Could you check a few things on this model? Use its own coordinates, in mm. A direction names the side the tool comes from. Round coordinates to 2 decimals unless told otherwise and drop trailing zeros. Loops run counter-clockwise (first coordinate to the right, second up) from the corner with the lowest first, then second, coordinate; pieces in that order, holes last. Notation, with made-up numbers: (40.5, 18) -> (92.5, 18) arc R32 ccw to (92.5, 50) -> close; hole circle Ø5 at (62.5, -23.5). An arc over 180 degrees is marked (long way). One line per item, written item: value.
from build123d import *

# Parameters (mm, degrees)
SKETCH1_R           = 27.5
SKETCH1_R_2         = 25
BOSS_EXTRUDE1_DEPTH = 100
SKETCH1_4_R         = 25
BOSS_EXTRUDE2_DEPTH = 175
BOSS_EXTRUDE4_START = 95
SKETCH6_R           = 27.5
SKETCH6_R_2         = 25
BOSS_EXTRUDE4_DEPTH = 95
BOSS_EXTRUDE5_START = 90
SKETCH8_R           = 25
BOSS_EXTRUDE5_DEPTH = 90
CUT_EXTRUDE1_START  = -115.215
CUT_EXTRUDE1_DEPTH  = 100.215
CUT_EXTRUDE3_START  = -40
SKETCH10_R          = 25
CUT_EXTRUDE3_DEPTH  = 40
CUT_EXTRUDE4_START  = 20
SKETCH11_R          = 25
SKETCH11_R_2        = 23.5
CUT_EXTRUDE4_DEPTH  = 3.4


with BuildPart() as part:
    # Sketch1 → Boss-Extrude1 (new, symmetric)
    # profile 1 of 2: a face of its own
    with BuildSketch(Plane(origin=(0, 0, 0), x_dir=(0, 0, -1), z_dir=(1, 0, 0))):
        Circle(SKETCH1_R)
        Circle(SKETCH1_R_2, mode=Mode.SUBTRACT)
    # profile 2 of 2: a face of its own
    with BuildSketch(Plane(origin=(0, 0, 0), x_dir=(0, 0, -1), z_dir=(1, 0, 0))):
        Circle(SKETCH1_R_2)
    extrude(amount=BOSS_EXTRUDE1_DEPTH, both=True)

    # Sketch1_4 → Boss-Extrude2 (add, symmetric)
    with BuildSketch(Plane(origin=(0, 0, 0), x_dir=(0, 0, -1), z_dir=(1, 0, 0))):
        Circle(SKETCH1_4_R)
    extrude(amount=BOSS_EXTRUDE2_DEPTH, both=True)

    # Sketch6 → Boss-Extrude4 (add)
    with BuildSketch(Plane(origin=(100, 0, 0), x_dir=(0, 0, -1), z_dir=(1, 0, 0)).offset(BOSS_EXTRUDE4_START)):
        Circle(SKETCH6_R)
        Circle(SKETCH6_R_2, mode=Mode.SUBTRACT)
    extrude(amount=-BOSS_EXTRUDE4_DEPTH)

    # Sketch8 → Boss-Extrude5 (add)
    with BuildSketch(Plane(origin=(175, 0, 0), x_dir=(0, 0, -1), z_dir=(1, 0, 0)).offset(BOSS_EXTRUDE5_START)):
        Circle(SKETCH8_R)
    extrude(amount=-BOSS_EXTRUDE5_DEPTH)

    # Sketch3 → Cut-Revolve1 (revolve, cut)
    with BuildSketch(Plane.XY, mode=Mode.PRIVATE) as cut_revolve1_sk:
        with BuildLine():
            Line((195, 25), (197, 25))
            ThreePointArc((197, 25), (196, 24), (195, 25))
        make_face()
        with BuildLine():
            Line((-100, 25), (-102, 25))
            ThreePointArc((-102, 25), (-101, 24), (-100, 25))
        make_face()
    revolve(cut_revolve1_sk.sketch.rotate(Axis((-100, 0, 0), (1, 0, 0)), 90), axis=Axis((-100, 0, 0), (1, 0, 0)), mode=Mode.SUBTRACT)

    # Sketch4 → Cut-Extrude1 (cut)
    with BuildSketch(Plane.ZY.offset(100).offset(CUT_EXTRUDE1_START)):
        with BuildLine():
            Line((-8, 26.310644234), (-8, 22.1))
            ThreePointArc((-8, 22.1), (-7.912132034, 21.887867966), (-7.7, 21.8))
            Line((-7.7, 21.8), (7.7, 21.8))
            ThreePointArc((7.7, 21.8), (7.912132034, 21.887867966), (8, 22.1))
            Line((8, 22.1), (8, 26.310644234))
            ThreePointArc((8, 26.310644234), (0, 27.5), (-8, 26.310644234))
        make_face()
    extrude(amount=CUT_EXTRUDE1_DEPTH, mode=Mode.SUBTRACT)

    # Sketch10 → Cut-Extrude3 (cut)
    with BuildSketch(Plane.ZY.offset(175).offset(CUT_EXTRUDE3_START)):
        Circle(SKETCH10_R)
    extrude(amount=CUT_EXTRUDE3_DEPTH, mode=Mode.SUBTRACT)

    # Sketch11 → Cut-Extrude4 (cut)
    with BuildSketch(Plane.ZY.offset(100).offset(CUT_EXTRUDE4_START)):
        Circle(SKETCH11_R)
        Circle(SKETCH11_R_2, mode=Mode.SUBTRACT)
    extrude(amount=CUT_EXTRUDE4_DEPTH, mode=Mode.SUBTRACT)


solid = part.part
(1) For faces 4 (the face through (-121.7, 7.1, 22.4)), 5 (the face through (-34, 21.8, 0)), 6 (the face through (-129.119, 7.509, -23.846)), which set-ups out of +Z, -Z, +X, -X, +Y, -Y let a thin tool reach every point of the face, with its end or its side?
Recorded:
face 4: none
face 5: +Y
face 6: -X
(2) I'm going to push flat-ended pins straight in: pin 1 Ø1.5 at (x, z) = (-3, 6) entering from -Y; pin 2 Ø2 at (x, y) = (58, 20.5) entering from -Z; pin 3 Ø5 at (x, z) = (73, -19) entering from -Y. Where does each tip first touch, or does it pass through?
Recorded:
pin 1: y = -26.99
pin 2: z = -19.39
pin 3: y = -22
(3) If we section it at C-C, the plane x = -65.5: Please give me the cut outline in (y, z).
Recorded:
outline: (21.8, -7.7) -> (21.8, 7.7) arc R0.3 cw to (22.1, 8) -> (26.31, 8) arc R27.5 ccw (long way) to (26.31, -8) -> (22.1, -8) arc R0.3 cw to start
(4) If we section it at B-B, the plane y = 0: Please give me the cut outline in (x, z), then the cut area to 3 significant figures.
Recorded:
outline: (-135, -25) -> (-123.4, -25) -> (-123.4, -23.5) -> (-120, -23.5) -> (-120, -25) -> (-102, -25) arc R1 cw to (-100, -25) -> (-100, -27.5) -> (195, -27.5) -> (195, -25) arc R1 cw to (197, -25) -> (265, -25) -> (265, 25) -> (197, 25) arc R1 cw to (195, 25) -> (195, 27.5) -> (-100, 27.5) -> (-100, 25) arc R1 cw to (-102, 25) -> (-120, 25) -> (-120, 23.5) -> (-123.4, 23.5) -> (-123.4, 25) -> (-135, 25) -> close
area: 21,500 mm²
(5) If we section it at D-D, the plane x = 204.5: Please give me the cut outline in (y, z), then the cut area to 3 significant figures.
Recorded:
outline: circle Ø50 at (0, 0)
area: 1,960 mm²
(6) If I drill on L1, parallel to X at y = -12, z = 21; L2, parallel to Z at x = 43.5, y = 1.5; L3, parallel to Z at x = 12, y = -2, over which ranges is the centre line in solid material (lowest first)?
Recorded:
L1: -135 to -123.4, -120 to -101.58, -100.42 to 195.42, 196.58 to 265
L2: -27.46 to 27.46
L3: -27.43 to 27.43
(7) If we section it at A-A, the plane z = 0: Please give me the cut outline in (x, y) (3 decimals).
Recorded:
outline: (-135, -25) -> (-123.4, -25) -> (-123.4, -23.5) -> (-120, -23.5) -> (-120, -25) -> (-102, -25) arc R1 cw to (-100, -25) -> (-100, -27.5) -> (195, -27.5) -> (195, -25) arc R1 cw to (197, -25) -> (265, -25) -> (265, 25) -> (197, 25) arc R1 cw to (195, 25) -> (195, 27.5) -> (15.215, 27.5) -> (15.215, 21.8) -> (-85, 21.8) -> (-85, 27.5) -> (-100, 27.5) -> (-100, 25) arc R1 cw to (-102, 25) -> (-120, 25) -> (-120, 23.5) -> (-123.4, 23.5) -> (-123.4, 25) -> (-135, 25) -> close
(8) Thinking about a two-plate mould opening in X: for faces 1 (the face through (-110.874, 7.509, -23.846)), 2 (the face through (195, -22.3, -12.1)), 3 (the face through (-123.4, -17, -17)), which applies, released by +X, released by -X, zero draft, split by the parting line, or undercut?
Recorded:
face 1: zero draft
face 2: released by +X
face 3: undercut
